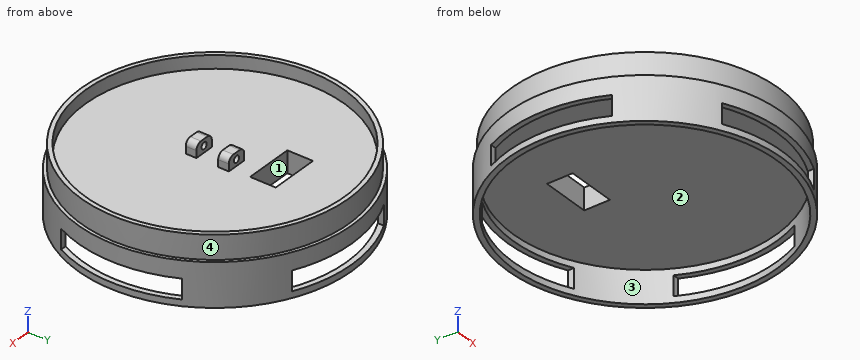
Solid Edge part; units mm, degrees
sketch "Sketch1" plane through (0, 0, 0) normal (0, 0, 1) x (1, 0, 0)
  line L0 (-15.0761, 2.2218) -> (-15.0761, 52.2218)
  line L1 (-15.0761, 52.2218) -> (-57.5761, 52.2218)
  line L2 (-57.5761, 52.2218) -> (-57.5761, 2.2218)
  line L3 (-57.5761, 2.2218) -> (-15.0761, 2.2218)
  line L4 (-25.0761, 30.4218) -> (-25.0761, 42.2218)
  line L5 (-25.0761, 42.2218) -> (-47.5761, 42.2218)
  line L6 (-47.5761, 42.2218) -> (-47.5761, 30.4218)
  line L7 (-47.5761, 30.4218) -> (-25.0761, 30.4218)
extrude "Protrusion1" add sketch "Sketch1" against normal blind 10
sketch "Sketch2" plane through (0, 0, 0) normal (0, 0, 1) x (1, 0, 0)
  line L0 (-23.2755, 17.1218) -> (-23.2755, 22.0207)
  line L1 (-23.2755, 22.0207) -> (-32.5481, 22.0207)
  line L2 (-32.5481, 22.0207) -> (-32.5481, 17.1218)
  line L3 (-32.5481, 17.1218) -> (-23.2755, 17.1218)
  line L4 (-23.2755, 7.1218) -> (-23.2755, 2.2218)
  line L5 (-23.2755, 2.2218) -> (-32.5481, 2.2218)
  line L6 (-32.5481, 2.2218) -> (-32.5481, 7.1218)
  line L7 (-32.5481, 7.1218) -> (-23.2755, 7.1218)
extrude "ExtrudedProtrusion_3" add sketch "Sketch2" along normal blind 6
sketch "Sketch3" plane through (-27.9118, 22.0207, 3) normal (0, 1, 0) x (1, 0, 0)
  circle A0 centre (0, 0) radius 1.55
extrude "ExtrudedCutout_1" cut sketch "Sketch3" against normal blind 17.5849
sketch "Sketch4" plane through (0, 0, 0) normal (0, 0, 1) x (1, 0, 0)
  circle A0 centre (-27.9118, 12.1218) radius 61.5
extrude "ExtrudedProtrusion_4" add sketch "Sketch4" against normal blind 10
sketch "Sketch5" plane through (0, 0, 0) normal (0, 0, 1) x (1, 0, 0)
  line L0 (-47.5761, 42.2218) -> (-47.5761, 30.4218)
  line L1 (-47.5761, 30.4218) -> (-25.0761, 30.4218)
  line L2 (-25.0761, 30.4218) -> (-25.0761, 42.2218)
  line L3 (-25.0761, 42.2218) -> (-47.5761, 42.2218)
extrude "ExtrudedCutout_2" cut sketch "Sketch5" against normal blind 44.8908
sketch "Sketch6" plane through (-27.9118, 12.1218, -5) normal (0, 0, -1) x (0, 1, 0)
  circle A0 centre (0, 0) radius 60.5
  circle A1 centre (0, 0) radius 63
extrude "ExtrudedProtrusion_6" add sketch "Sketch6" along normal blind 20
sketch "Sketch7" plane through (-27.9118, -50.8782, -15) normal (0, -1, 0) x (0, 0, 1)
  line L0 (-7.0569, 27.7607) -> (2.0569, 27.7607)
  line L1 (2.0569, 27.7607) -> (2.0569, -27.7607)
  line L2 (2.0569, -27.7607) -> (-7.0569, -27.7607)
  line L3 (-7.0569, -27.7607) -> (-7.0569, 27.7607)
extrude "ExtrudedCutout_3" cut sketch "Sketch7" against normal blind 172.1374
pattern_circular "Pattern_1" count 4 over 360 about axis through (-27.9118, 12.1218, -25) along (0, 0, 1) of "ExtrudedCutout_3"
sketch "Sketch8" plane through (-27.9118, 12.1218, 0) normal (0, 0, 1) x (0, -1, 0)
  circle A0 centre (0, 0) radius 59.5
  circle A1 centre (0, 0) radius 61.5
extrude "Protrusion2" add sketch "Sketch8" along normal blind 6
fillet "Round_1" radius 2.75 4 edges at (-32.5481, 4.6718, 6) (-23.2755, 4.6718, 6) (-32.5481, 19.5713, 6) (-23.2755, 19.5713, 6)
The model under review builds one solid part; all positions refer to its coordinate system, in mm. Face numbers are marked on the shaded views. A direction names the side the tool comes from. Round coordinates to 2 decimals unless told otherwise and drop trailing zeros. Loops run counter-clockwise (first coordinate to the right, second up) from the corner with the lowest first, then second, coordinate; pieces in that order, holes last. Notation, with made-up numbers: (13, 86) -> (59, 86) arc R32 cw to (59, 114) -> close; hole circle Ø9 at (-2.5, -30.75). An arc over 180 degrees is marked (long way). Return JSON: item names as keys, results as strings.
(1) For the marked faces 1 and 2, list the 3-axis set-ups (+Z, -Z, +X, -X, +Y, -Y) from which the entire face can be reached by the end or side of a thin tool; tool diameter is ignored.
Solved:
{"face 1": "+Z, -Z", "face 2": "-Z"}
(2) Add section D-D on y = 62. Write out the cut boundary in (x, z), plus the area to 3 significant figures.
Solved:
{"outline": "(-66.4, -25) -> (-62.15, -25) -> (-62.15, -10) -> (6.33, -10) -> (6.33, -25) -> (10.57, -25) -> (10.57, -5) -> (8.07, -5) -> (8.07, 6) -> (4.53, 6) -> (4.53, 0) -> (-60.35, 0) -> (-60.35, 6) -> (-63.89, 6) -> (-63.89, -5) -> (-66.4, -5) -> close", "area": "914 mm2"}
(3) For line 1 (X direction, y = 18.15, z = 3); line 2 (X direction, y = 5.8, z = 3) (1 decimal); line 3 (Z direction, x = -21, y = 42), list the stretches that pass through material, from the lowest coordinate up.
Solved:
{"line 1": "-89.12 to -87.11, -32.55 to -29.46, -26.36 to -23.28, 31.28 to 33.29", "line 2": "-89.1 to -87.1, -32.5 to -29.5, -26.4 to -23.3, 31.3 to 33.3", "line 3": "-10 to 0"}
(4) The part is to be moulded in two halves that separate along X. For the marked faces 3 and 4, say which applies: released by +X, released by -X, zero draft, split by the parting line, or undercut.
Solved:
{"face 3": "undercut", "face 4": "split by the parting line"}
(5) For pin 1 (0.8 mm diameter, centred on x = -83, z = -17, fed in from +Y); pin 2 (6 mm diameter, centred on x = -67, z = -8, fed in from +Y); pin 3 (8 mm diameter, centred on x = -32, z = -3, fed in from +Y), all flat-tipped, find the tip position at first contact; note any pin that passes through.
Solved:
{"pin 1": "y = 43.4", "pin 2": "y = 63.76", "pin 3": "y = 75.12"}
(6) Add section C-C on x = -61. Write out the cut boundary in (y, z).
Solved:
{"outline": "(-41.49, -25) -> (-38.53, -25) -> (-38.53, -10) -> (62.77, -10) -> (62.77, -25) -> (65.73, -25) -> (65.73, -5) -> (63.96, -5) -> (63.96, 6) -> (61.57, 6) -> (61.57, 0) -> (-37.33, 0) -> (-37.33, 6) -> (-39.72, 6) -> (-39.72, -5) -> (-41.49, -5) -> close"}
(7) Add section A-A on z = -20. Write out the cut boundary in (x, y).
Solved:
{"outline": "(-84.47, -15.64) arc R63 ccw to (-55.67, -44.43) -> (-55.67, -41.63) arc R60.5 cw to (-81.67, -15.64) -> close; (-84.47, 39.88) -> (-81.67, 39.88) arc R60.5 cw to (-55.67, 65.88) -> (-55.67, 68.68) arc R63 ccw to start; (-0.15, -44.43) arc R63 ccw to (28.64, -15.64) -> (25.84, -15.64) arc R60.5 cw to (-0.15, -41.63) -> close; (-0.15, 65.88) arc R60.5 cw to (25.84, 39.88) -> (28.64, 39.88) arc R63 ccw to (-0.15, 68.68) -> close"}
